from build123d import *

# Parameters (mm, degrees)
SKETCH1_W               = 8
SKETCH1_H               = 8
BOSS_EXTRUDE1_DEPTH     = 3
CUT_EXTRUDE1_DEPTH      = 12.704699911
CUT_EXTRUDE1_DEPTH_BACK = 12.704699911
CUT_EXTRUDE2_DEPTH      = 11
SKETCH4_R               = 1.8
CUT_EXTRUDE3_DEPTH      = 0.8
SKETCH5_W               = 8
SKETCH5_H               = 1
BOSS_EXTRUDE2_DEPTH     = 2
FILLET1_R               = 4
CUT_EXTRUDE4_DEPTH      = 0.4
CUT_EXTRUDE5_DEPTH      = 0.4


with BuildPart() as part:
    # Sketch1 → Boss-Extrude1 (new body)
    with BuildSketch(Plane(origin=(0, 0, 0), x_dir=(1, 0, 0), z_dir=(0, 1, 0))):
        with Locations((4, 4)):
            Rectangle(SKETCH1_W, SKETCH1_H)
    extrude(amount=BOSS_EXTRUDE1_DEPTH)

    # Sketch2 → Cut-Extrude1 (cut, two sides: drawn at the far end of the back side and taken through both)
    with BuildSketch(Plane.XY.offset(-CUT_EXTRUDE1_DEPTH_BACK)):
        Polygon((0, 0), (0.6, 3), (0, 3), align=None)
        Polygon((8, 0), (7.4, 3), (8, 3), align=None)
    extrude(amount=CUT_EXTRUDE1_DEPTH + CUT_EXTRUDE1_DEPTH_BACK, mode=Mode.SUBTRACT)

    # Sketch3 → Cut-Extrude2 (cut)
    with BuildSketch(Plane(origin=(0, 0, 0), x_dir=(0, 0, -1), z_dir=(1, 0, 0))):
        Polygon((0, 0), (0.6, 3), (0, 3), align=None)
        Polygon((8, 3), (7.4, 3), (8, 0), align=None)
    extrude(amount=CUT_EXTRUDE2_DEPTH, mode=Mode.SUBTRACT)

    # Sketch4 → Cut-Extrude3 (cut)
    with BuildSketch(Plane.XZ):
        with Locations(Location((4, -3.75, 0), (0, 0, 270))):
            Circle(SKETCH4_R)
    extrude(amount=-CUT_EXTRUDE3_DEPTH, mode=Mode.SUBTRACT)

    # Sketch5 → Boss-Extrude2 (add)
    with BuildSketch(Plane.XZ):
        with Locations((4, -7.5)):
            Rectangle(SKETCH5_W, SKETCH5_H)
    extrude(amount=BOSS_EXTRUDE2_DEPTH)

    # Fillet1
    # the kernel refuses this fillet: 4 mm, written as the material it takes off along each edge
    with BuildSketch(Plane(origin=(8, -2, -16.660254038), x_dir=(0, 1, 0), z_dir=(0, 0, 1)), Plane(origin=(0, -2, 1.660254038), x_dir=(0, 1, 0), z_dir=(0, 0, -1))) as fillet1_piece_1:
        with BuildLine():
            CenterArc((4, 3.464101615), FILLET1_R, 180, 60)
            Line((0, 3.464101615), (-0.08, 3.464101615))
            Line((-0.08, 3.464101615), (-0.08, 0))
            Line((-0.08, 0), (0, -0.08))
            ThreePointArc((0, -0.08), (1, -0.08), (1.96, -0.069282032))
            Line((1.96, -0.069282032), (2, 0))
        make_face()
    extrude(amount=18.320508076, mode=Mode.SUBTRACT)

    # Sketch6 → Cut-Extrude4 (cut)
    with BuildSketch(Plane(origin=(0, 3, 0), x_dir=(1, 0, 0), z_dir=(0, 1, 0))):
        with BuildLine():
            Line((4.053794593, 3.505457585), (4.053794593, 4.172124252))
            Line((4.053794593, 4.172124252), (5.797384337, 4.172124252))
            Line((5.797384337, 4.172124252), (5.797384337, 2.564752457))
            add(Edge.make_bspline(
                [(5.797384337, 2.564752457), (5.775440275, 2.544992361), (5.730582172, 2.504598726), (5.657391115, 2.447633596), (5.576814656, 2.393249062), (5.489339896, 2.340343698), (5.394785806, 2.289343315), (5.293529517, 2.239537607), (5.185384208, 2.19141366), (5.032450931, 2.131128575), (4.835594452, 2.065533422), (4.594933471, 2.008496304), (4.352368706, 1.973513189), (4.190125473, 1.969167013), (4.109083055, 1.966996047)],
                knots=[0, 0, 0, 0, 0.581799769, 1.189316438, 1.825828404, 2.496525428, 3.203088405, 3.942228803, 4.719818701, 5.534979611, 7.181138583, 8.803804008, 10.403462225, 12, 12, 12, 12], degree=3))
            add(Edge.make_bspline(
                [(4.109083055, 1.966996047), (4.058312627, 1.967758979), (3.958229013, 1.969262944), (3.810482794, 1.981368296), (3.667847904, 2.002080495), (3.530208107, 2.031409962), (3.397097502, 2.066765974), (3.26907094, 2.111868039), (3.146582956, 2.166009466), (3.028523806, 2.226338905), (2.917094396, 2.295632176), (2.812187083, 2.371432832), (2.714561168, 2.454400196), (2.624566637, 2.544701507), (2.540998329, 2.641714843), (2.464831298, 2.745902822), (2.396526155, 2.857385727), (2.335239765, 2.974765127), (2.280716867, 3.097008702), (2.234709094, 3.223154334), (2.194374003, 3.351370526), (2.161222966, 3.482107416), (2.136875151, 3.615790052), (2.117947657, 3.751799892), (2.107781758, 3.890986734), (2.105984472, 3.984609884), (2.105076645, 4.031899893)],
                knots=[0, 0, 0, 0, 1.124918047, 2.217548049, 3.282233239, 4.316494221, 5.334437038, 6.332151046, 7.320712088, 8.300141923, 9.267552434, 10.225301062, 11.165776911, 12.103230934, 13.047553934, 14.000517593, 14.959782875, 15.941944936, 16.932894943, 17.923491392, 18.915624898, 19.910402922, 20.909870877, 21.92519501, 22.95199481, 24, 24, 24, 24], degree=3))
            add(Edge.make_bspline(
                [(2.105076645, 4.031899893), (2.105812881, 4.082940857), (2.107264322, 4.183564655), (2.119773705, 4.33228546), (2.139199297, 4.476648194), (2.168656936, 4.616390773), (2.20449512, 4.75216369), (2.248233589, 4.883877531), (2.301822866, 5.010556427), (2.361436063, 5.133283761), (2.429297714, 5.250362339), (2.505977563, 5.360290437), (2.589206445, 5.464176802), (2.680629029, 5.560371285), (2.779923369, 5.648827012), (2.886080088, 5.730522243), (2.998844963, 5.806865303), (3.079553832, 5.849911113), (3.120301004, 5.871643482)],
                knots=[0, 0, 0, 0, 1.105010302, 2.178452875, 3.229459892, 4.257086284, 5.268538906, 6.268935615, 7.259234261, 8.24469117, 9.221745683, 10.185929258, 11.144249683, 12.101504986, 13.055838221, 14.020611351, 15.000673771, 16, 16, 16, 16], degree=3))
            add(Edge.make_bspline(
                [(3.120301004, 5.871643482), (3.152638085, 5.887700047), (3.218317351, 5.920312247), (3.322813337, 5.959248923), (3.432101667, 5.994677516), (3.547832356, 6.021111591), (3.6692195, 6.042829226), (3.796209305, 6.059036287), (3.929210312, 6.067547239), (4.019595582, 6.068879104), (4.065813824, 6.069560149)],
                knots=[0, 0, 0, 0, 0.887969848, 1.803539625, 2.741143579, 3.713741423, 4.722068772, 5.775476617, 6.8624965, 8, 8, 8, 8], degree=3))
            add(Edge.make_bspline(
                [(4.065813824, 6.069560149), (4.125403824, 6.06867255), (4.241295356, 6.066946335), (4.410256532, 6.05256252), (4.569271079, 6.027772487), (4.718560435, 5.993629866), (4.857802985, 5.949731518), (4.986759025, 5.895763799), (5.106220057, 5.832812796), (5.214455834, 5.758355608), (5.313666102, 5.676257846), (5.403591975, 5.586419647), (5.48426965, 5.488707943), (5.555752499, 5.383614392), (5.617477906, 5.2707046), (5.670549966, 5.151008328), (5.714234697, 5.023616882), (5.73534656, 4.935145779), (5.746102286, 4.89007297)],
                knots=[0, 0, 0, 0, 1.271135529, 2.472123572, 3.614091059, 4.701890498, 5.736279567, 6.724681829, 7.680621489, 8.611506429, 9.52200816, 10.424540711, 11.318996785, 12.221421405, 13.131851814, 14.060431888, 15.011860567, 16, 16, 16, 16], degree=3))
            Line((5.746102286, 4.89007297), (4.976871517, 4.736226816))
            add(Edge.make_bspline(
                [(4.976871517, 4.736226816), (4.969254672, 4.761468809), (4.95422678, 4.81127079), (4.925094227, 4.882758251), (4.891539922, 4.949961192), (4.853483379, 5.013366036), (4.810541206, 5.072582433), (4.761675926, 5.126971617), (4.709961453, 5.179014495), (4.652020351, 5.225088646), (4.590259767, 5.266624284), (4.52537561, 5.304078684), (4.455901775, 5.334453158), (4.382811411, 5.358892727), (4.306461756, 5.37964837), (4.225856415, 5.392413169), (4.141900573, 5.402040295), (4.084540473, 5.402606041), (4.055397158, 5.402893482)],
                knots=[0, 0, 0, 0, 1.027736275, 2.027704492, 3.005900071, 3.954421694, 4.908588141, 5.853155543, 6.803277083, 7.766271258, 8.734041521, 9.704274878, 10.683578894, 11.68490234, 12.708089448, 13.76461009, 14.864251086, 16, 16, 16, 16], degree=3))
            add(Edge.make_bspline(
                [(4.055397158, 5.402893482), (4.01128773, 5.401716629), (3.925204424, 5.399419898), (3.799534269, 5.384433236), (3.680976007, 5.357770589), (3.569219615, 5.320994553), (3.46406021, 5.273789934), (3.366918824, 5.2143961), (3.275376693, 5.146327474), (3.192038786, 5.066438045), (3.116460773, 4.976859168), (3.051034483, 4.876522357), (2.996567377, 4.765751945), (2.951955713, 4.645104141), (2.91643531, 4.514573915), (2.892338718, 4.373699188), (2.876594443, 4.222696077), (2.875085403, 4.118480819), (2.874307414, 4.064752457)],
                knots=[0, 0, 0, 0, 1.043810997, 2.037086103, 2.989314757, 3.91471467, 4.817033861, 5.710208705, 6.603920097, 7.511448416, 8.435617211, 9.371747005, 10.338444094, 11.350425613, 12.411431869, 13.5347293, 14.729025275, 16, 16, 16, 16], degree=3))
            add(Edge.make_bspline(
                [(2.874307414, 4.064752457), (2.875118698, 4.00702506), (2.876695474, 3.894828493), (2.892027057, 3.732262921), (2.917247643, 3.580803592), (2.95342224, 3.44064155), (2.998941149, 3.311279521), (3.053656914, 3.192304252), (3.121182779, 3.085923464), (3.197244894, 2.990004781), (3.28225913, 2.906191636), (3.37384152, 2.833121051), (3.471482188, 2.77119638), (3.576081527, 2.721395085), (3.686320303, 2.681751972), (3.80321198, 2.653959398), (3.926408504, 2.636695674), (4.010734238, 2.634687946), (4.053794593, 2.633662713)],
                knots=[0, 0, 0, 0, 1.318042826, 2.561693173, 3.724929596, 4.821196409, 5.862977565, 6.853497791, 7.804600806, 8.73339865, 9.643480846, 10.524649628, 11.404635349, 12.277659519, 13.165160235, 14.075017549, 15.017020959, 16, 16, 16, 16], degree=3))
            add(Edge.make_bspline(
                [(4.053794593, 2.633662713), (4.097408334, 2.634875039), (4.185053042, 2.637311287), (4.316328539, 2.657956024), (4.448117665, 2.68833542), (4.577327471, 2.734163302), (4.70281192, 2.786727561), (4.819965055, 2.847306941), (4.929675356, 2.910453005), (4.995733738, 2.959668979), (5.028153568, 2.98382297)],
                knots=[0, 0, 0, 0, 0.993821502, 1.997150276, 3.023717651, 4.073291794, 5.118404464, 6.123376694, 7.078999408, 8, 8, 8, 8], degree=3))
            Line((5.028153568, 2.98382297), (5.028153568, 3.505457585))
            Line((5.028153568, 3.505457585), (4.053794593, 3.505457585))
        make_face()
    extrude(amount=-CUT_EXTRUDE4_DEPTH, mode=Mode.SUBTRACT)

    # Sketch7 → Cut-Extrude5 (cut)
    with BuildSketch(Plane(origin=(0, 3, 0), x_dir=(1, 0, 0), z_dir=(0, 1, 0))):
        Polygon((7.051946272, 3.224540865), (7.051946272, 0.93992548), (6.405792426, 0.93992548), (6.405792426, 1.23992548), (6.705792426, 1.23992548), (6.705792426, 2.924540865), (6.405792426, 2.924540865), (6.405792426, 3.224540865), align=None)
    extrude(amount=-CUT_EXTRUDE5_DEPTH, mode=Mode.SUBTRACT)


solid = part.part
Here's how the part is built. I have some questions about the finished solid (model axes, mm). A direction names the side the tool comes from. Round coordinates to 2 decimals unless told otherwise and drop trailing zeros. Loops run counter-clockwise (first coordinate to the right, second up) from the corner with the lowest first, then second, coordinate; pieces in that order, holes last. Notation, with made-up numbers: (-1.75, 24) - (14.25, 24) arc R27 ccw to (14.25, 54) - close; hole circle Ø6 at (40, 82). An arc over 180 degrees is marked (long way). One line per question, with ' | ' between items. Start each with the question number.
Q1. I want a section at B-B (z = -1.5). Write out the boundary of the cut face in (x, y), then the cut area to 3 significant figures.
Q2. I want a section at C-C (y = 2). Write out the boundary of the cut face in (x, z), then the cut area to 3 significant figures.
Q3. Will these pins go through, and if not, where does the flat tip stop? pin 1 (1.5 mm diameter, centred on x = 2, y = 1, fed in from +Z); pin 2 (4.5 mm diameter, centred on x = 4, z = -3.75, fed in from -Y); pin 3 (1.1 mm diameter, centred on x = 3, z = -3.5, fed in from -Y).
Q4. We'd pull the mould along X, two halves only. Please class faces 4 (the cylindrical face through (1.49, -1.48, -7.49)), 5 (the flat face through (4, 0.8, -4)), 6 (the cylindrical face through (6.51, -1.48, -7.51)), 7 (the flat face through (3.2, 3, -4)): +X half, -X half, draft (parallel to the pull), parting line (faces both ways), or undercut.
Q5. For faces 1 (the flat face through (4, -1, -8)), 2 (the cylindrical face through (4.541, 0.394, -5.467)), 3 (the flat face through (4, -1, -7)), which set-ups out of +Z, -Z, +X, -X, +Y, -Y let a thin tool reach every point of the face, with its end or its side?
Q6. I want a section at D-D (y = 1.4). Write out the boundary of the cut face in (x, z), then the cut area to 3 significant figures.
Q7. I want a section at A-A (y = 0.1). Write out the boundary of the cut face in (x, z).
Q8. Please list where these lines run through material, in increasing order: line 1 (Y direction, x = 3.5, z = -3.5); line 2 (Y direction, x = 5.25, z = -3); line 3 (X direction, y = 0.2, z = -3.75). Write a range as [from, to].
Response values:
1) outline: (0, 0) - (8, 0) - (7.4, 3) - (7.05, 3) - (7.05, 2.6) - (6.71, 2.6) - (6.71, 3) - (0.6, 3) - close | area: 22.1 mm²
2) outline: (0.4, -7.6) - (7.6, -7.6) - (7.6, -0.4) - (0.4, -0.4) - close | area: 51.8 mm²
3) pin 1: stops at z = -0.05 | pin 2: stops at y = 0 | pin 3: stops at y = 0.8
4) face 4: -X half | face 5: undercut | face 6: +X half | face 7: draft
5) face 1: -Z, +X, -X, +Y, -Y | face 2: -Y | face 3: +Z, +X, -X, -Y
6) outline: (0.28, -7.72) - (7.72, -7.72) - (7.72, -0.28) - (0.28, -0.28) - close | area: 55.4 mm²
7) outline: (0.02, -7.98) - (7.98, -7.98) - (7.98, -0.02) - (0.02, -0.02) - close; hole circle Ø3.6 at (4, -3.75)
8) line 1: y = [0.8, 3] | line 2: y = [0.8, 2.6] | line 3: x = [0.04, 2.2], [5.8, 7.96]
